CAD build for the part. Positions are in the model's coordinates, mm. A direction names the side the tool comes from. Coordinates: 2 decimals unless noted, no trailing zeros. Write each loop counter-clockwise with the first axis right and the second up, starting at its lowest first coordinate (ties: lowest second). Pieces come first, ordered by that corner, then holes. Notation, with made-up numbers: (25, 36.25) - (76, 36.25) arc R30 cw to (76, 71.25) - close; hole circle Ø11 at (26, -13). An arc over 180 degrees is marked (long way). Answer in a Markdown table with one row per item. Add a question column.
Q1. Band-saw the part on C-C (x = 1). List the corners of the cut face in (y, z).
Q2. Band-saw the part on A-A (y = -23.5). List the corners of the cut face in (x, z), and give its area (3 significant figures).
Q3. Band-saw the part on D-D (x = -13). List the corners of the cut face in (y, z).
Q4. Two-plate mould, pull along X, no slides. Class faces 4 (the flat face through (0, -6, 1)), 5 (the cylindrical face through (32.995, -24.1, -7.395)), 6 (the flat face through (-32, -23, -15)), 7 (the cylindrical face through (-7.587, 10.668, 0.986)): +X half, -X half, draft (parallel to the pull), parting line (faces both ways), or undercut.
Q5. Pin check, flat tips, straight feed: pin 1 (2 mm diameter, centred on y = -8.5, z = 1.5, fed in from -X); pin 2 (1 mm diameter, centred on y = -22.5, z = 1, fed in from -X); pin 3 (2 mm diameter, centred on y = 1.5, z = -12.5, fed in from -X); pin 4 (12 mm diameter, centred on x = 24.5, y = -37, fed in from -Z). Stop position of each tip, or through.
Q6. Band-saw the part on B-B (z = -2). List the corners of the cut face in (x, y), and give its area (3 significant figures).
Q7. 3-axis set-ups, long thin cutter, end or side, ignore diameter. For faces 1 (the flat face through (0, -39, 0)), 2 (the cylindrical face through (-32.995, -22.9, -7.395)), 3 (the flat face through (0, -32, 1)): which of +Z, -Z, +X, -X, +Y, -Y reach the whole face in a straight line?
Q8. Drill centre lines: line 1 along Y through (x, z) = (0, 1.4); line 2 along X through (y, z) = (-24, -1.25); line 3 along Z through (x, y) = (17, -5.5). Where is each one in solid material? Low to high. Write a range as from..to.
Autodesk Inventor part; units mm, degrees
ref_plane "Work Plane1" through (0, 0, 0) normal (0, 0, 1) x (1, 0, 0)
ref_plane "YZ Plane" through (0, 0, 0) normal (1, 0, 0) x (0, 1, 0)
ref_plane "XZ Plane" through (0, 0, 0) normal (0, 1, 0) x (-1, 0, 0)
sketch "Sketch1" plane through (0, 0, 0) normal (0, 0, 1) x (1, 0, 0)
  arc A0 (8.8357, -55.2951) -> (8.8357, 8.2951) centre (0, -23.5) ccw
  arc A1 (-8.8357, 8.2951) -> (-8.8357, -55.2951) centre (0, -23.5) ccw
  arc A2 (-8.4341, 6.8499) -> (-8.4341, -53.8499) centre (0, -23.5) ccw
  arc A3 (8.4341, -53.8499) -> (8.4341, 6.8499) centre (0, -23.5) ccw
  line L0 (-8.4341, 6.8499) -> (-8.8357, 8.2951)
  line L1 (-8.4341, -53.8499) -> (-8.8357, -55.2951)
  line L2 (8.4341, -53.8499) -> (8.8357, -55.2951)
  line L3 (8.8357, 8.2951) -> (8.4341, 6.8499)
  dimension "d36" = 1.5
  dimension "d37" = 1.5
extrude "Extrusion1" add sketch "Sketch1" against normal blind 15
ref_plane "Work Plane1" through (0, 0, 0) normal (0, 0, 1) x (1, 0, 0)
sketch "Sketch2" plane through (0, 0, 0) normal (0, 0, 1) x (1, 0, 0)
  circle A0 centre (0, -23.5) radius 35
  circle A1 centre (0, 5) radius 1.5
  circle A2 centre (0, -52) radius 1.5
  circle A3 centre (0, 5) radius 2
  circle A4 centre (0, -52) radius 2
  line L0 (-25, -11) -> (25, -11)
  line L1 (25, -11) -> (25, -36)
  line L2 (25, -36) -> (-25, -36)
  line L3 (-25, -36) -> (-25, -11)
  line L4 (-25, -11) -> (25, -36) construction
  line L5 (25, -11) -> (-25, -36) construction
  line L6 (-19, -32) -> (19, -32)
  line L7 (19, -32) -> (19, -15)
  line L8 (19, -15) -> (-19, -15)
  line L9 (-19, -15) -> (-19, -32)
  line L10 (-19, -32) -> (19, -15) construction
  line L11 (19, -32) -> (-19, -15) construction
  line L12 (5, -18) -> (-5, -18)
  line L13 (-5, -18) -> (-5, -6)
  line L14 (-5, -6) -> (5, -6)
  line L15 (5, -6) -> (5, -18)
  line L16 (5, -18) -> (-5, -6) construction
  line L17 (-5, -18) -> (5, -6) construction
  point P0 (0, 0)
  point P1 (-5, -11)
  point P2 (0, -12)
  point P3 (5, -15)
  point P4 (-5, -15)
  dimension "d4" = 4
  dimension "d5" = 4
  dimension "d38" = 50
  dimension "d39" = 25
  dimension "d40" = 38
  dimension "d41" = 17
  dimension "d44" = 10
  dimension "d45" = 12
  dimension "d46" = 7
extrude "Extrusion2" add sketch "Sketch2" along normal blind 2 contours A0 | L0 L13 L8 L9 L6 L7 L15 L1 L2 L3
properties part number "lid2"
Checked values:
| question | item | result |
|---|---|---|
| 1 | outline | (-58.49, 0) - (-53.73, 0) - (-53.73, 2) - (-58.49, 2) - close; (-50.27, 0) - (-32, 0) - (-32, 2) - (-50.27, 2) - close; (-6, 0) - (3.27, 0) - (3.27, 2) - (-6, 2) - close; (6.73, 0) - (11.49, 0) - (11.49, 2) - (6.73, 2) - close |
| 2 | outline | (-35, 0) - (-33, 0) - (-33, -15) - (-31.5, -15) - (-31.5, 0) - (-19, 0) - (-19, 2) - (-35, 2) - close; (19, 0) - (31.5, 0) - (31.5, -15) - (33, -15) - (33, 0) - (35, 0) - (35, 2) - (19, 2) - close |
| 2 | area | 109 mm² |
| 3 | outline | (-56, 0) - (-53.83, 0) - (-53.83, -15) - (-52.19, -15) - (-52.19, 0) - (-32, 0) - (-32, 2) - (-56, 2) - close; (-15, 0) - (5.19, 0) - (5.19, -15) - (6.83, -15) - (6.83, 0) - (9, 0) - (9, 2) - (-15, 2) - close |
| 4 | face 4 | undercut |
| 4 | face 5 | +X half |
| 4 | face 6 | draft |
| 4 | face 7 | parting line |
| 5 | pin 1 | stops at x = -32.08 |
| 5 | pin 2 | stops at x = -35 |
| 5 | pin 3 | stops at x = -22.65 |
| 5 | pin 4 | stops at z = -15 |
| 6 | outline | (-8.84, -55.3) - (-8.43, -53.85) arc R31.5 cw to (-8.43, 6.85) - (-8.84, 8.3) arc R33 ccw to start; (8.43, -53.85) - (8.84, -55.3) arc R33 ccw to (8.84, 8.3) - (8.43, 6.85) arc R31.5 cw to start |
| 6 | area | 251 mm² |
| 7 | face 1 | -Z |
| 7 | face 2 | -Z, -X |
| 7 | face 3 | +Z, -Z |
| 8 | line 1 | y = -58.5..-54, -50..-32, -6..3, 7..11.5 |
| 8 | line 2 | x = -33..-31.5, 31.5..33 |
| 8 | line 3 | z = 0..2 |
